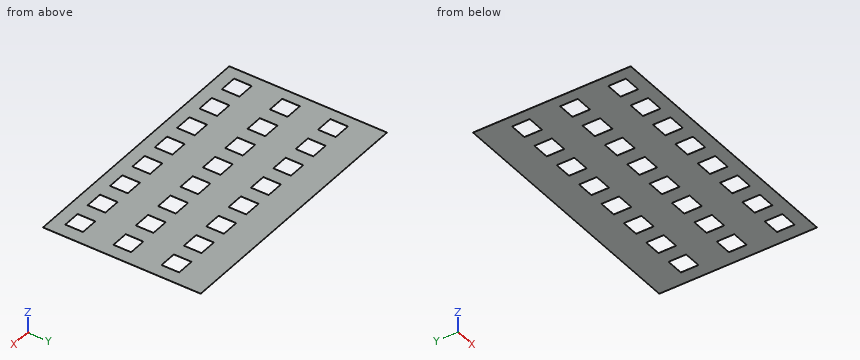
```python
from build123d import *

# Parameters (mm, degrees)
MODEL_W             = 1870
MODEL_H             = 1180
BASE_FLANGE1_DEPTH  = 0.6
TAB1_DEPTH          = 0.6
SKETCH7_W           = 65
SKETCH7_H           = 1180
TAB2_DEPTH          = 0.6
SKETCH9_W           = 1840.328960488
SKETCH9_H           = 1045.942358838
BOSS_EXTRUDE1_DEPTH = 0.6
SKETCH8_W           = 132
SKETCH8_H           = 132
CUT_EXTRUDE1_DEPTH  = 10


# Sheet-metal steps are written as plain solids
with BuildPart() as part:
    # Model → Base-Flange1 (new body)
    with BuildSketch(Plane.XY):
        with Locations((935, 590)):
            Rectangle(MODEL_W, MODEL_H)
        Polygon((1790, 440), (1640, 440), (1640, 595), (1650, 595), (1650, 662), (1780, 662), (1780, 595), (1790, 595), align=None, mode=Mode.SUBTRACT)
        Polygon((1595, 440), (1445, 440), (1445, 595), (1455, 595), (1455, 662), (1585, 662), (1585, 595), (1595, 595), align=None, mode=Mode.SUBTRACT)
        Polygon((1400, 440), (1250, 440), (1250, 595), (1260, 595), (1260, 662), (1390, 662), (1390, 595), (1400, 595), align=None, mode=Mode.SUBTRACT)
        Polygon((1205, 440), (1055, 440), (1055, 595), (1065, 595), (1065, 662), (1195, 662), (1195, 595), (1205, 595), align=None, mode=Mode.SUBTRACT)
        Polygon((1010, 440), (860, 440), (860, 595), (870, 595), (870, 662), (1000, 662), (1000, 595), (1010, 595), align=None, mode=Mode.SUBTRACT)
        Polygon((815, 440), (665, 440), (665, 595), (675, 595), (675, 662), (805, 662), (805, 595), (815, 595), align=None, mode=Mode.SUBTRACT)
        Polygon((620, 440), (470, 440), (470, 595), (480, 595), (480, 662), (610, 662), (610, 595), (620, 595), align=None, mode=Mode.SUBTRACT)
        Polygon((425, 440), (275, 440), (275, 595), (285, 595), (285, 662), (415, 662), (415, 595), (425, 595), align=None, mode=Mode.SUBTRACT)
        Polygon((230, 440), (80, 440), (80, 595), (90, 595), (90, 662), (220, 662), (220, 595), (230, 595), align=None, mode=Mode.SUBTRACT)
        Polygon((1790, 805), (1640, 805), (1640, 960), (1650, 960), (1650, 1027), (1780, 1027), (1780, 960), (1790, 960), align=None, mode=Mode.SUBTRACT)
        Polygon((1595, 805), (1445, 805), (1445, 960), (1455, 960), (1455, 1027), (1585, 1027), (1585, 960), (1595, 960), align=None, mode=Mode.SUBTRACT)
        Polygon((1400, 805), (1250, 805), (1250, 960), (1260, 960), (1260, 1027), (1390, 1027), (1390, 960), (1400, 960), align=None, mode=Mode.SUBTRACT)
        Polygon((1205, 805), (1055, 805), (1055, 960), (1065, 960), (1065, 1027), (1195, 1027), (1195, 960), (1205, 960), align=None, mode=Mode.SUBTRACT)
        Polygon((1010, 805), (860, 805), (860, 960), (870, 960), (870, 1027), (1000, 1027), (1000, 960), (1010, 960), align=None, mode=Mode.SUBTRACT)
        Polygon((815, 805), (665, 805), (665, 960), (675, 960), (675, 1027), (805, 1027), (805, 960), (815, 960), align=None, mode=Mode.SUBTRACT)
        Polygon((620, 805), (470, 805), (470, 960), (480, 960), (480, 1027), (610, 1027), (610, 960), (620, 960), align=None, mode=Mode.SUBTRACT)
        Polygon((425, 805), (275, 805), (275, 960), (285, 960), (285, 1027), (415, 1027), (415, 960), (425, 960), align=None, mode=Mode.SUBTRACT)
        Polygon((230, 805), (80, 805), (80, 960), (90, 960), (90, 1027), (220, 1027), (220, 960), (230, 960), align=None, mode=Mode.SUBTRACT)
        Polygon((1790, 75), (1640, 75), (1640, 230), (1650, 230), (1650, 297), (1780, 297), (1780, 230), (1790, 230), align=None, mode=Mode.SUBTRACT)
        Polygon((1595, 75), (1445, 75), (1445, 230), (1455, 230), (1455, 297), (1585, 297), (1585, 230), (1595, 230), align=None, mode=Mode.SUBTRACT)
        Polygon((1400, 75), (1250, 75), (1250, 230), (1260, 230), (1260, 297), (1390, 297), (1390, 230), (1400, 230), align=None, mode=Mode.SUBTRACT)
        Polygon((1205, 75), (1055, 75), (1055, 230), (1065, 230), (1065, 297), (1195, 297), (1195, 230), (1205, 230), align=None, mode=Mode.SUBTRACT)
        Polygon((1010, 75), (860, 75), (860, 230), (870, 230), (870, 297), (1000, 297), (1000, 230), (1010, 230), align=None, mode=Mode.SUBTRACT)
        Polygon((815, 75), (665, 75), (665, 230), (675, 230), (675, 297), (805, 297), (805, 230), (815, 230), align=None, mode=Mode.SUBTRACT)
        Polygon((620, 75), (470, 75), (470, 230), (480, 230), (480, 297), (610, 297), (610, 230), (620, 230), align=None, mode=Mode.SUBTRACT)
        Polygon((425, 75), (275, 75), (275, 230), (285, 230), (285, 297), (415, 297), (415, 230), (425, 230), align=None, mode=Mode.SUBTRACT)
        Polygon((230, 75), (80, 75), (80, 230), (90, 230), (90, 297), (220, 297), (220, 230), (230, 230), align=None, mode=Mode.SUBTRACT)
    extrude(amount=-BASE_FLANGE1_DEPTH)

    # Sketch6 → Tab1 (add)
    with BuildSketch(Plane.XY):
        Polygon((1705, 805), (1725, 805), (1725, 806), (1789, 806), (1789, 959), (1779, 959), (1779, 1026), (1725, 1026), (1725, 1027), (1705, 1027), (1705, 1026), (1651, 1026), (1651, 959), (1641, 959), (1641, 806), (1705, 806), align=None)
        Polygon((1705, 440), (1725, 440), (1725, 441), (1789, 441), (1789, 594), (1779, 594), (1779, 661), (1725, 661), (1725, 662), (1705, 662), (1705, 661), (1651, 661), (1651, 594), (1641, 594), (1641, 441), (1705, 441), align=None)
        Polygon((1705, 75), (1725, 75), (1725, 76), (1789, 76), (1789, 229), (1779, 229), (1779, 296), (1725, 296), (1725, 297), (1705, 297), (1705, 296), (1651, 296), (1651, 229), (1641, 229), (1641, 76), (1705, 76), align=None)
    extrude(amount=-TAB1_DEPTH)

    # Sketch7 → Tab2 (add)
    with BuildSketch(Plane.XY):
        with Locations((1902.5, 590)):
            Rectangle(SKETCH7_W, SKETCH7_H)
        with Locations((-32.5, 590)):
            Rectangle(SKETCH7_W, SKETCH7_H)
    extrude(amount=-TAB2_DEPTH)

    # Sketch9 → Boss-Extrude1 (add)
    with BuildSketch(Plane.XY):
        with Locations((950.64470062, 555.573524784)):
            Rectangle(SKETCH9_W, SKETCH9_H)
    extrude(amount=-BOSS_EXTRUDE1_DEPTH)

    # Sketch8 → Cut-Extrude1 (cut)
    with BuildSketch(Plane.XY):
        with Locations((1767.05073242, 881.911611336)):
            Rectangle(SKETCH8_W, SKETCH8_H)
        with Locations((1527.05073242, 881.911611336)):
            Rectangle(SKETCH8_W, SKETCH8_H)
        with Locations((1287.05073242, 881.911611336)):
            Rectangle(SKETCH8_W, SKETCH8_H)
        with Locations((1047.05073242, 881.911611336)):
            Rectangle(SKETCH8_W, SKETCH8_H)
        with Locations((807.05073242, 881.911611336)):
            Rectangle(SKETCH8_W, SKETCH8_H)
        with Locations((567.05073242, 881.911611336)):
            Rectangle(SKETCH8_W, SKETCH8_H)
        with Locations((327.05073242, 881.911611336)):
            Rectangle(SKETCH8_W, SKETCH8_H)
        with Locations((87.05073242, 881.911611336)):
            Rectangle(SKETCH8_W, SKETCH8_H)
        with Locations((1527.05073242, 521.911611336)):
            Rectangle(SKETCH8_W, SKETCH8_H)
        with Locations((1287.05073242, 521.911611336)):
            Rectangle(SKETCH8_W, SKETCH8_H)
        with Locations((1047.05073242, 521.911611336)):
            Rectangle(SKETCH8_W, SKETCH8_H)
        with Locations((807.05073242, 521.911611336)):
            Rectangle(SKETCH8_W, SKETCH8_H)
        with Locations((567.05073242, 521.911611336)):
            Rectangle(SKETCH8_W, SKETCH8_H)
        with Locations((327.05073242, 521.911611336)):
            Rectangle(SKETCH8_W, SKETCH8_H)
        with Locations((87.05073242, 521.911611336)):
            Rectangle(SKETCH8_W, SKETCH8_H)
        with Locations((1527.05073242, 161.911611336)):
            Rectangle(SKETCH8_W, SKETCH8_H)
        with Locations((1287.05073242, 161.911611336)):
            Rectangle(SKETCH8_W, SKETCH8_H)
        with Locations((1047.05073242, 161.911611336)):
            Rectangle(SKETCH8_W, SKETCH8_H)
        with Locations((807.05073242, 161.911611336)):
            Rectangle(SKETCH8_W, SKETCH8_H)
        with Locations((567.05073242, 161.911611336)):
            Rectangle(SKETCH8_W, SKETCH8_H)
        with Locations((327.05073242, 161.911611336)):
            Rectangle(SKETCH8_W, SKETCH8_H)
        with Locations((87.05073242, 161.911611336)):
            Rectangle(SKETCH8_W, SKETCH8_H)
        with Locations((1767.05073242, 521.911611336)):
            Rectangle(SKETCH8_W, SKETCH8_H)
        with Locations((1767.05073242, 161.911611336)):
            Rectangle(SKETCH8_W, SKETCH8_H)
    extrude(amount=-CUT_EXTRUDE1_DEPTH, mode=Mode.SUBTRACT)


solid = part.part
```
Read the model definition and answer for the solid it produces. Units are mm, in the model's axes. Coordinates: 2 decimals unless noted, no trailing zeros. Loops run counter-clockwise (first coordinate to the right, second up) from the corner with the lowest first, then second, coordinate; pieces in that order, holes last. Notation, with made-up numbers: (22, 5.5) -> (58, 5.5) arc R23 cw to (58, 21.5) -> close; hole circle Ø9 at (10.5, 22). An arc over 180 degrees is marked (long way). Return JSON: item names as keys, results as strings.
Item 1: Find the intervals of material crossed by probe 1 along Y at (x, z) = (1805.5, -0.15), in increasing order.
Answers:
{"probe 1": "y = 0 to 95.91, 227.91 to 455.91, 587.91 to 815.91, 947.91 to 1180"}
Item 2: Find section A-A (x = 66.5). Determine the outline of the cut face in (y, z), plus the area to 3 significant figures.
Answers:
{"outline": "(0, -0.6) -> (95.91, -0.6) -> (95.91, 0) -> (0, 0) -> close; (227.91, -0.6) -> (455.91, -0.6) -> (455.91, 0) -> (227.91, 0) -> close; (587.91, -0.6) -> (815.91, -0.6) -> (815.91, 0) -> (587.91, 0) -> close; (947.91, -0.6) -> (1180, -0.6) -> (1180, 0) -> (947.91, 0) -> close", "area": "470 mm2"}
Item 3: A flat-ended cylindrical pin translates along its axis: P1, Ø1.5, axis at x = 1437, y = 473, coming from the +Z side. Find the tip coordinate at first contact, or state that the pin passes through.
Answers:
{"P1": "stops at z = 0"}
Item 4: Find section B-B (z = -0.4). Count the separate pieces of the cut face and the enclosed holes in it, plus the area to 3 significant figures.
Answers:
{"separate pieces": "1", "enclosed holes": "24", "area": "1,940,000 mm2"}
